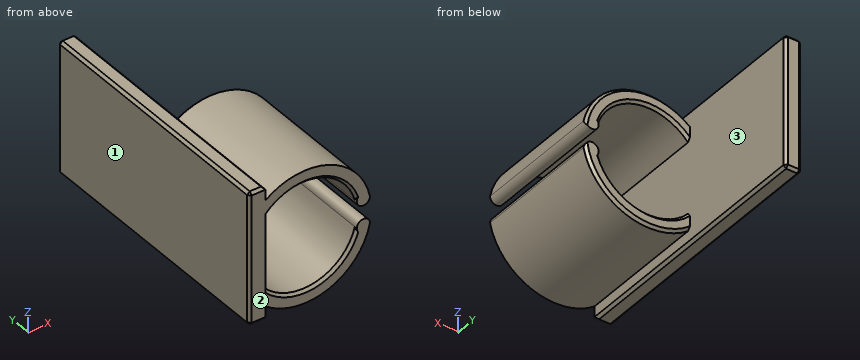
from build123d import *

# Parameters (mm, degrees)
SKETCH001_W     = 2.5
SKETCH001_H     = 40
PAD001_DEPTH    = 20
PAD002_DEPTH    = 20
CHAMFER001_SIZE = 0.4


with BuildPart() as part:
    # Sketch001 → Pad001 (new body)
    with BuildSketch(Plane.XY):
        with Locations((18.401947, 24.9952)):
            Rectangle(SKETCH001_W, SKETCH001_H)
    extrude(amount=PAD001_DEPTH)

    # Sketch002 (on Face4 of Pad001) → Pad002 (join)
    with BuildSketch(Plane.XZ.offset(-4.9952)):
        with BuildLine():
            ThreePointArc((35.449906, 12), (29.202457, 19.348469), (19.651947, 18))
            Line((19.651947, 18), (19.651947, 15.367324))
            ThreePointArc((33.449906, 12), (27.56058, 17.820824), (19.651947, 15.367324))
            ThreePointArc((33.449906, 12), (34.449906, 11), (35.449906, 12))
        make_face()
        with BuildLine():
            ThreePointArc((19.651947, 2), (29.202457, 0.651531), (35.449906, 8))
            ThreePointArc((35.449906, 8), (34.449906, 9), (33.449906, 8))
            ThreePointArc((19.651947, 4.632676), (27.56058, 2.179176), (33.449906, 8))
            Line((19.651947, 4.632676), (19.651947, 2))
        make_face()
    extrude(amount=-PAD002_DEPTH)

    # Chamfer001
    chamfer001_edges = [part.edges().sort_by_distance(p)[0] for p in [
        (19.651947, 24.9952, 20),
        (18.401947, 44.9952, 20),
        (17.151947, 24.9952, 20),
        (18.401947, 4.9952, 20),
        (19.651947, 24.9952, 0),
        (18.401947, 44.9952, 0),
        (17.151947, 24.9952, 0),
        (18.401947, 4.9952, 0),
        (19.651947, 44.9952, 10),
        (17.151947, 44.9952, 10),
        (17.151947, 4.9952, 10),
        (29.202457, 24.9952, 19.348469),
        (29.202457, 24.9952, 0.651531),
        (27.56058, 24.9952, 17.820824),
        (27.56058, 24.9952, 2.179176),
        (27.56058, 4.9952, 17.820824),
        (27.56058, 4.9952, 2.179176),
    ]]
    chamfer(chamfer001_edges, length=CHAMFER001_SIZE)


solid = part.part
Geometry: final body of the model. Coordinates: model frame, mm. Face numbers are marked on the shaded views. Give positions to 0.01 mm unless a question says otherwise; leave off trailing zeros. Loops run counter-clockwise (first coordinate to the right, second up) from the corner with the lowest first, then second, coordinate; pieces in that order, holes last. Notation, with made-up numbers: (69.5, 46) - (125.5, 46) arc R27 cw to (125.5, 65) - close; hole circle Ø1 at (85.5, -16). An arc over 180 degrees is marked (long way). One line per question, with ' | ' between items. Start each with the question number.
(1) Section query B-B on y = 17.5. Return loops of the section in (x, z), then the cut area to 3 significant figures.
(2) Contact query for flat-ended pins moving along their axis: pin 1 (6 mm diameter, centred on x = 21.5, z = 3, fed in from +Y); pin 2 (9.5 mm diameter, centred on x = 30, z = 6.5, fed in from +Y); pin 3 (3 mm diameter, centred on x = 30.5, y = 19.5, fed in from -Z). Output: stop coordinate, or through.
(3) Section query A-A on y = 31. Return loops of the section in (x, z).
(4) Ray query, line 1 (X direction, y = 30, z = 2.5); line 2 (Z direction, x = 20.5, y = 16); line 3 (Z direction, x = 27.5, y = 24). Return the intervals inside material, ascending. Write a range as from..to.
(5) Pull-direction query (X, two-part tool) for the marked faces 1, 2 and 3; classes: released by +X, released by -X, zero draft, split by the parting line, or undercut.
The answers:
1) outline: (17.15, 0.4) - (17.55, 0) - (19.25, 0) - (19.65, 0.4) - (19.65, 2) arc R10 ccw to (35.45, 8) arc R1 ccw to (33.45, 8) arc R8.05 cw to (19.65, 4.63) - (19.65, 15.37) arc R8.05 cw to (33.45, 12) arc R1 ccw to (35.45, 12) arc R10 ccw to (19.65, 18) - (19.65, 19.6) - (19.25, 20) - (17.55, 20) - (17.15, 19.6) - close | area: 126 mm2
2) pin 1: y = 45 | pin 2: y = 25 | pin 3: z = 0.58
3) outline: (17.15, 0.4) - (17.55, 0) - (19.25, 0) - (19.65, 0.4) - (19.65, 19.6) - (19.25, 20) - (17.55, 20) - (17.15, 19.6) - close
4) line 1: 17.15..19.65 | line 2: 1.43..3.81, 16.19..18.57 | line 3: 0.17..2.16, 17.84..19.83
5) face 1: released by -X | face 2: zero draft | face 3: undercut
